The listing builds one solid part. Answer for the finished solid, in the listing's coordinates (mm). A direction names the side the tool comes from. Round coordinates to 2 decimals unless told otherwise and drop trailing zeros. Loops run counter-clockwise (first coordinate to the right, second up) from the corner with the lowest first, then second, coordinate; pieces in that order, holes last. Notation, with made-up numbers: M -32.5,-22.75 L -13.5,-22.75 A22 cw -13.5,-8.75 Z; hole C -4.5,69 d10. An arc over 180 degrees is marked long. Put each result on its own line as item: value. Start each with the question number.
(1) Straight lines are drawn through the part: line 1 (Y direction, x = 52.5, z = -1.2); line 2 (Z direction, x = 4, y = 17); line 3 (Y direction, x = 59, z = 53.5). For each, find the intervals that lie inside material, in ascending order.
(2) Section A-A, the plane x = 22.5 is taken. Determine the outline of the cut face in (y, z), then the cut area to 3 significant figures.
(3) Section B-B, the plane x = 58.5 is taken. Determine the outline of the cut face in (y, z), then the cut area to 3 significant figures.
(4) Section D-D, the plane z = 67.5 is taken. Determine the outline of the cut face in (x, y).
(5) Flat-ended cylindrical pins translate along their axes: P1, Ø4, axis at x = 51, y = 20, coming from the +Z side; P2, Ø8, axis at x = 23.5, z = 49, coming from the +Y side. Find the tip coordinate at first contact, or state that the pin passes through.
(6) Which of the six approach directions +Z, -Z, +X, -X, +Y, -Y give full straight-line access (tool end or side, diameter ignored) to faces 1 (the face through (37, 2, 37)), 2 (the face through (37, 42, -2))?
(7) Section C-C, the plane y = 54.5 is taken. Determine the outline of the cut face in (x, z).
(8) Determine the mould class of faces 3 (the face through (75, 22.4, -0.4)), 4 (the face through (22.825, 73.845, -1.014)), 5 (the face through (37, 80, -1)) for opening direction Y: released by +Y, released by -Y, zero draft, split by the parting line, or undercut.
```python
from build123d import *

# Parameters (mm, degrees)
SKETCH2_W                    = 75
SKETCH2_H                    = 80
BASE_FLANGE1_DEPTH           = 2
EDGE_FLANGE1_STRIP_W         = 9.4732
EDGE_FLANGE1_STRIP_H         = 2
EDGE_FLANGE1_STRIP_CUT_DEPTH = 75
EDGE_FLANGE1_DEPTH           = 75
CUT_EXTRUDE1_REACH           = 134.853
SKETCH10_R                   = 2.5


# Sheet-metal steps are written as plain solids
with BuildPart() as part:
    # Sketch2 → Base-Flange1 (new body)
    with BuildSketch(Plane.XY):
        with Locations((37.5, 40)):
            Rectangle(SKETCH2_W, SKETCH2_H)
    extrude(amount=-BASE_FLANGE1_DEPTH)

    # Edge-Flange1 strip (across the edge) → Edge-Flange1 strip cut (cut)
    with BuildSketch(Plane.YZ):
        with Locations((-2, -1)):
            Rectangle(EDGE_FLANGE1_STRIP_W, EDGE_FLANGE1_STRIP_H)
    extrude(amount=EDGE_FLANGE1_STRIP_CUT_DEPTH, mode=Mode.SUBTRACT)

    # Edge-Flange1 section (across the edge) → Edge-Flange1 (add)
    with BuildSketch(Plane.YZ):
        with BuildLine():
            Line((0, 0.7366), (0, 73))
            Line((0, 73), (2, 73))
            Line((2, 73), (2, 0.7366))
            ThreePointArc((2, 0.7366), (2.215745145, 0.215745145), (2.7366, 0))
            Line((2.7366, 0), (2.7366, -2))
            ThreePointArc((2.7366, -2), (0.801531583, -1.198468417), (0, 0.7366))
        make_face()
    extrude(amount=EDGE_FLANGE1_DEPTH)

    # Sketch10 → Cut-Extrude1 (cut, up to next)
    with BuildSketch(Plane(origin=(0, 0, -2), x_dir=(-1, 0, 0), z_dir=(0, 0, -1)), mode=Mode.PRIVATE) as cut_extrude1_sk1:
        with Locations((-22.5, 11.37)):
            Circle(SKETCH10_R)
    cut_extrude1_tool1 = extrude(cut_extrude1_sk1.sketch, amount=-CUT_EXTRUDE1_REACH, mode=Mode.PRIVATE) & part.part
    # Sketch10 → Cut-Extrude1 (cut, up to next)
    with BuildSketch(Plane(origin=(0, 0, -2), x_dir=(-1, 0, 0), z_dir=(0, 0, -1)), mode=Mode.PRIVATE) as cut_extrude1_sk2:
        with Locations((-52.5, 71.37)):
            Circle(SKETCH10_R)
    cut_extrude1_tool2 = extrude(cut_extrude1_sk2.sketch, amount=-CUT_EXTRUDE1_REACH, mode=Mode.PRIVATE) & part.part
    # Sketch10 → Cut-Extrude1 (cut, up to next)
    with BuildSketch(Plane(origin=(0, 0, -2), x_dir=(-1, 0, 0), z_dir=(0, 0, -1)), mode=Mode.PRIVATE) as cut_extrude1_sk3:
        with Locations((-52.5, 11.3666)):
            Circle(SKETCH10_R)
    cut_extrude1_tool3 = extrude(cut_extrude1_sk3.sketch, amount=-CUT_EXTRUDE1_REACH, mode=Mode.PRIVATE) & part.part
    # Sketch10 → Cut-Extrude1 (cut, up to next)
    with BuildSketch(Plane(origin=(0, 0, -2), x_dir=(-1, 0, 0), z_dir=(0, 0, -1)), mode=Mode.PRIVATE) as cut_extrude1_sk4:
        with Locations((-22.5, 71.3666)):
            Circle(SKETCH10_R)
    cut_extrude1_tool4 = extrude(cut_extrude1_sk4.sketch, amount=-CUT_EXTRUDE1_REACH, mode=Mode.PRIVATE) & part.part
    add(cut_extrude1_tool1.solids().sort_by_distance((22.5, 11.37, -2))[0], mode=Mode.SUBTRACT)
    add(cut_extrude1_tool2.solids().sort_by_distance((52.5, 71.37, -2))[0], mode=Mode.SUBTRACT)
    add(cut_extrude1_tool3.solids().sort_by_distance((52.5, 11.3666, -2))[0], mode=Mode.SUBTRACT)
    add(cut_extrude1_tool4.solids().sort_by_distance((22.5, 71.3666, -2))[0], mode=Mode.SUBTRACT)


solid = part.part
```
Recorded:
1. line 1: y = 0.8 to 8.87, 13.87 to 68.87, 73.87 to 80
1. line 2: z = -2 to 0
1. line 3: y = 0 to 2
2. outline: M 0,0.74 A2.74 ccw 2.74,-2 L 8.87,-2 L 8.87,0 L 2.74,0 A0.74 cw 2,0.74 L 2,73 L 0,73 Z; M 13.87,-2 L 68.87,-2 L 68.87,0 L 13.87,0 Z; M 73.87,-2 L 80,-2 L 80,0 L 73.87,0 Z
2. area: 285 mm²
3. outline: M 0,0.74 A2.74 ccw 2.74,-2 L 80,-2 L 80,0 L 2.74,0 A0.74 cw 2,0.74 L 2,73 L 0,73 Z
3. area: 305 mm²
4. outline: M 0,0 L 75,0 L 75,2 L 0,2 Z
5. P1: stops at z = 0
5. P2: stops at y = 2
6. face 1: +Z, +X, -X, +Y
6. face 2: -Z, +X, -X, +Y, -Y
7. outline: M 0,-2 L 75,-2 L 75,0 L 0,0 Z
8. face 3: zero draft
8. face 4: undercut
8. face 5: released by +Y
